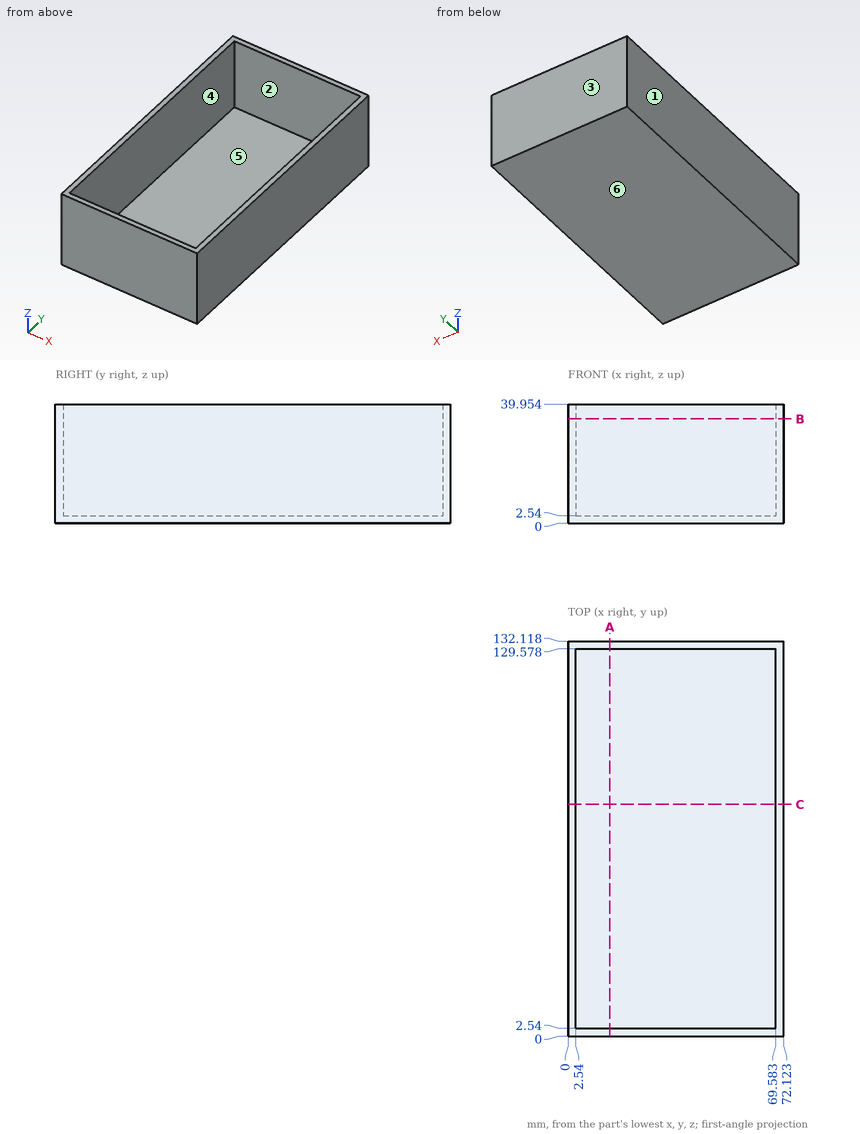
Print and shaded views of the part. All mm, measured from the part's lowest x, y and z. A direction names the side the tool comes from. Round coordinates to 2 decimals unless told otherwise and drop trailing zeros. Write each loop counter-clockwise with the first axis right and the second up, starting at its lowest first coordinate (ties: lowest second). Pieces come first, ordered by that corner, then holes.
Item 1: Cut at B-B, the plane z = 35. Give the cut face in (x, y), plus the area to 3 significant figures.
Results:
outline: (0, 0) - (72.12, 0) - (72.12, 132.12) - (0, 132.12) - close; hole (2.54, 2.54) - (69.58, 2.54) - (69.58, 129.58) - (2.54, 129.58) - close
area: 1,010 mm2
Item 2: Cut at A-A, the plane x = 14. Give the cut face in (y, z).
Results:
outline: (0, 0) - (132.12, 0) - (132.12, 39.95) - (129.58, 39.95) - (129.58, 2.54) - (2.54, 2.54) - (2.54, 39.95) - (0, 39.95) - close
Item 3: Cut at C-C, the plane y = 77.5. Give the cut face in (x, z).
Results:
outline: (0, 0) - (72.12, 0) - (72.12, 39.95) - (69.58, 39.95) - (69.58, 2.54) - (2.54, 2.54) - (2.54, 39.95) - (0, 39.95) - close
Item 4: Drop a flat-ended pin along its axis: pin 1 Ø6 at (x, z) = (17, 27) entering from -Y. Give the stop position or say it passes through.
Results:
pin 1: stops at y = 0
Item 5: Which spindle directions (+Z, -Z, +X, -X, +Y, -Y) get a long thin tool onto all of the face, cutting with end or side? Do the marked faces 1 and 2. Say none if no direction does.
Results:
face 1: +Z, -Z, -X, +Y, -Y
face 2: +Z
Item 6: Probe L1, parallel to X at y = 71, z = 35.5; L2, parallel to Y at x = 13.5, z = 31; L3, parallel to Z at x = 45.5, y = 26.5. List the from-to ranges inside material, lowest first.
Results:
L1: x = 0 to 2.54, 69.58 to 72.12
L2: y = 0 to 2.54, 129.58 to 132.12
L3: z = 0 to 2.54
Item 7: Two-plate mould, pull along Y, no slides. Class the marked faces 3, 4, 5 and 6: +Y half, -Y half, draft (parallel to the pull), parting line (faces both ways), or undercut.
Results:
face 3: +Y half
face 4: undercut
face 5: undercut
face 6: draft
